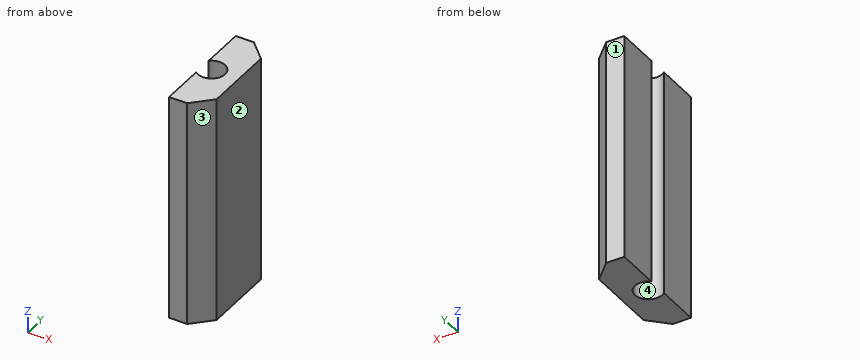
```python
from build123d import *

# Parameters (mm, degrees)
CYLINDER1144_R     = 1.5
CYLINDER1144_DEPTH = 50
BOX457_W           = 4
BOX457_H           = 12
BOX457_DEPTH       = 25
CHAMFER_SIZE       = 2


with BuildPart() as obj1:
    # Cylinder1144 → Cylinder1144 (new body)
    with BuildSketch(Plane(origin=(52, 0, 0), x_dir=(1, 0, 0), z_dir=(0, 0, 1))):
        Circle(CYLINDER1144_R)
    extrude(amount=CYLINDER1144_DEPTH)


with BuildPart() as cut428:
    # Box457 → Box457 (new body)
    with BuildSketch(Plane(origin=(51, -6, 20), x_dir=(1, 0, 0), z_dir=(0, 0, 1))):
        with Locations((2, 6)):
            Rectangle(BOX457_W, BOX457_H)
    extrude(amount=BOX457_DEPTH)

    # Chamfer
    chamfer_edges = [cut428.edges().sort_by_distance(p)[0] for p in [
        (55, -6, 32.5),
        (55, 6, 32.5),
    ]]
    chamfer(chamfer_edges, length=CHAMFER_SIZE)

    # Cut428: cut obj1
    add(obj1.part, mode=Mode.SUBTRACT)


solid = cut428.part
```
CAD build for the part. Positions are in the model's coordinates, mm. Face numbers are marked on the shaded views. Round coordinates to 2 decimals unless told otherwise and drop trailing zeros. Loops run counter-clockwise (first coordinate to the right, second up) from the corner with the lowest first, then second, coordinate; pieces in that order, holes last. Notation, with made-up numbers: (-2, 19.5) - (44, 19.5) arc R31 cw to (44, 56.5) - close; hole circle Ø10 at (42.5, 35.25). An arc over 180 degrees is marked (long way). Return JSON: item names as keys, results as strings. Group by question number.
Q1. Band-saw the part on D-D on x = 54.15. Give the cut face in (y, z), plus the area to 4 significant figures.
Q2. Band-saw the part on C-C on y = 0. Give the cut face in (x, z), plus the area to 3 significant figures.
Q3. Two-plate mould, pull along Y, no slides. Class the marked faces 1, 2, 3 and 4: +Y half, -Y half, draft (parallel to the pull), parting line (faces both ways), or undercut.
Q4. Drill centre lines: line 1 along Y through (x, z) = (52, 32.75); line 2 along X through (y, z) = (0, 33.75); line 3 along X through (y, z) = (5.5, 30). Where is each one in solid material? Low to high. Write a range as [from, to].
Q5. Band-saw the part on B-B on z = 43.75. Give the cut face in (x, y), plus the area to 3 significant figures.
Q6. Band-saw the part on A-A on x = 52. Give the cut face in (y, z), plus the area to 3 significant figures.
Solutions:
{
 "1": {"outline": "(-4.85, 20) - (4.85, 20) - (4.85, 45) - (-4.85, 45) - close", "area": "242.5 mm^2"},
 "2": {"outline": "(53.5, 20) - (55, 20) - (55, 45) - (53.5, 45) - close", "area": "37.5 mm^2"},
 "3": {"face 1": "+Y half", "face 2": "draft", "face 3": "-Y half", "face 4": "undercut"},
 "4": {"line 1": "y = [-6, -1.5], [1.5, 6]", "line 2": "x = [53.5, 55]", "line 3": "x = [51, 53.5]"},
 "5": {"outline": "(51, -6) - (53, -6) - (55, -4) - (55, 4) - (53, 6) - (51, 6) - (51, 1.12) arc R1.5 cw (long way) to (51, -1.12) - close", "area": "37.7 mm^2"},
 "6": {"outline": "(-6, 20) - (-1.5, 20) - (-1.5, 45) - (-6, 45) - close; (1.5, 20) - (6, 20) - (6, 45) - (1.5, 45) - close", "area": "225 mm^2"}
}
